```python
from build123d import *

# Parameters (mm, degrees)
CROQUIS1_W              = 40
CROQUIS1_H              = 40
CROQUIS1_W_2            = 36
CROQUIS1_H_2            = 36
SALIENTE_EXTRUIR1_DEPTH = 600
CORTAR_EXTRUIR2_DEPTH   = 41


with BuildPart() as part:
    # Croquis1 → Saliente-Extruir1 (new body)
    with BuildSketch(Plane(origin=(0, 0, 0), x_dir=(0, 0, -1), z_dir=(1, 0, 0))):
        Rectangle(CROQUIS1_W, CROQUIS1_H)
        Rectangle(CROQUIS1_W_2, CROQUIS1_H_2, mode=Mode.SUBTRACT)
    extrude(amount=SALIENTE_EXTRUIR1_DEPTH)

    # Croquis2 → Cortar-Extruir2 (cut, through all)
    with BuildSketch(Plane(origin=(0, 20, 0), x_dir=(1, 0, 0), z_dir=(0, 1, 0))):
        Polygon((0, 20), (0, -20), (40, -20), align=None)
        Polygon((560, -20), (600, 20), (600, -20), align=None)
    extrude(amount=-CORTAR_EXTRUIR2_DEPTH, mode=Mode.SUBTRACT)


solid = part.part
```
The listing builds one solid part. Answer for the finished solid, in the listing's coordinates (mm). A direction names the side the tool comes from. Round coordinates to 2 decimals unless told otherwise and drop trailing zeros. Loops run counter-clockwise (first coordinate to the right, second up) from the corner with the lowest first, then second, coordinate; pieces in that order, holes last.
Q1. Section C-C, the plane x = 543.5 is taken. Determine the outline of the cut face in (y, z).
Q2. Which of the six approach directions +Z, -Z, +X, -X, +Y, -Y give full straight-line access (tool end or side, diameter ignored) to faces 1 (the face through (296, 0, -18)), 2 (the face through (296, -20, 0))?
Q3. Section B-B, the plane y = 3.5 is taken. Determine the outline of the cut face in (x, z).
Q4. For a pull along Y with two mould halves and no side action, classify faces 3 (the face through (296, 20, 0)), 4 (the face through (296, 0, 18)), 5 (the face through (296, 0, -20)) as released by +Y, released by -Y, zero draft, split by the parting line, or undercut.
Q5. Find the intervals of material crossed by line 1 (Z direction, x = 203, y = -11), in increasing order.
Q6. Section A-A, the plane z = 6.5 is taken. Determine the outline of the cut face in (x, y).
Completed:
1. outline: (-20, -20) - (20, -20) - (20, 20) - (-20, 20) - close; hole (-18, -18) - (18, -18) - (18, 18) - (-18, 18) - close
2. face 1: +X, -X
2. face 2: +Z, -Z, +X, -X, -Y
3. outline: (0, -20) - (600, -20) - (598, -18) - (2, -18) - close; (38, 18) - (562, 18) - (560, 20) - (40, 20) - close
4. face 3: released by +Y
4. face 4: undercut
4. face 5: zero draft
5. line 1: z = -20 to -18, 18 to 20
6. outline: (26.5, -20) - (573.5, -20) - (573.5, -18) - (26.5, -18) - close; (26.5, 18) - (573.5, 18) - (573.5, 20) - (26.5, 20) - close
